Job drawing, mm, ordinate dimensions from the low corner. One solid piece. Give positions to 0.01 mm unless a question says otherwise; leave off trailing zeros. Write each loop counter-clockwise with the first axis right and the second up, starting at its lowest first coordinate (ties: lowest second). Pieces come first, ordered by that corner, then holes. Notation, with made-up numbers: M -27,49 L 26,49 A14 cw 26,57 Z; hole C 66.25,1.25 d3. An arc over 180 degrees is marked long. Answer as CSV lines item,"result". Start each with the question number.
Item 1: Band-saw the part on A-A, the plane y = 1.6. List the corners of the cut face in (x, z).
Item 2: Wall check: L1, parallel to X at y = 1.8, z = 4.5; L2, parallel to Z at x = 1.5, y = 0.6. Give the ranges that are in metal, low to high. Write a range as from..to.
Item 3: Pin check, flat tips, straight feed: pin 1 (0.6 mm diameter, centred on x = 1, y = 1.5, fed in from -Z); pin 2 (0.6 mm diameter, centred on x = 1, y = 1, fed in from +Z). Stop position of each tip, or through.
Item 4: Band-saw the part on B-B, the plane z = 22.5. List the corners of the cut face in (x, y).
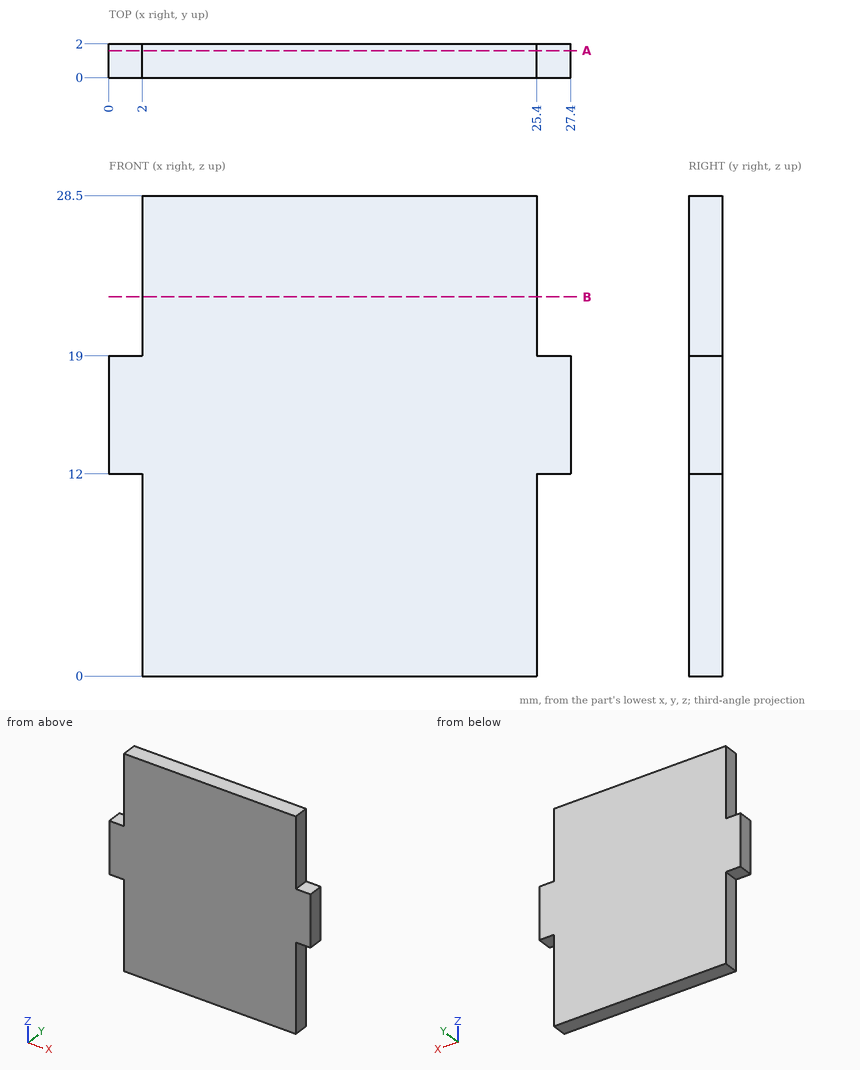
Output:
1,outline,"M 0,12 L 2,12 L 2,0 L 25.4,0 L 25.4,12 L 27.4,12 L 27.4,19 L 25.4,19 L 25.4,28.5 L 2,28.5 L 2,19 L 0,19 Z"
2,L1,"2..25.4"
2,L2,"12..19"
3,pin 1,"z = 12"
3,pin 2,"z = 19"
4,outline,"M 2,0 L 25.4,0 L 25.4,2 L 2,2 Z"
